Answer from the drawing. Dimensions are ordinates in mm from the lowest x, y and z of the part. A direction names the side the tool comes from. Round coordinates to 2 decimals unless told otherwise and drop trailing zeros. Order: outer loops, then holes, each group sorted by start corner. A loop starts at its lowest first (then second) coordinate and runs counter-clockwise, first axis right, second up. Notation, with made-up numbers: (12.25, 36.25) -> (67.25, 36.25) arc R17 cw to (67.25, 49.25) -> close; hole circle Ø8 at (32, 58.5). An arc over 180 degrees is marked (long way). Use a Markdown table: item, result. Add a question column.
Item 1: A flat-ended cylindrical pin translates along its axis: P1, Ø1, axis at x = 54, z = 20.5, coming from the +Y side. Find the tip coordinate at first contact, or state that the pin passes through.
Item 2: A cutting plane is placed at C-C, the plane x = 65.5. Determine the outline of the cut face in (y, z), plus the area to 3 significant figures.
Item 3: For a pull along Y with two mould halves and no side action, classify the marked faces 3, 4 and 5 as +Y half, -Y half, draft (parallel to the pull), parting line (faces both ways), or undercut.
Item 4: A tool of negligible diameter and unlimited length cuts with its end or side. For the marked faces 1 and 2, from which of +Z, -Z, +X, -X, +Y, -Y can it reach the whole face along a straight path? Write none if from no direction.
Item 5: A cutting plane is placed at B-B, the plane y = 71. Determine the outline of the cut face in (x, z), plus the area to 3 significant figures.
Item 6: Find the intervals of material crossed by L1, parallel to X at y = 55, z = 30.5; L2, parallel to Z at x = 6, y = 9; L3, parallel to X at y = 36, z = 25, in increasing order. Write a range as [from, to].
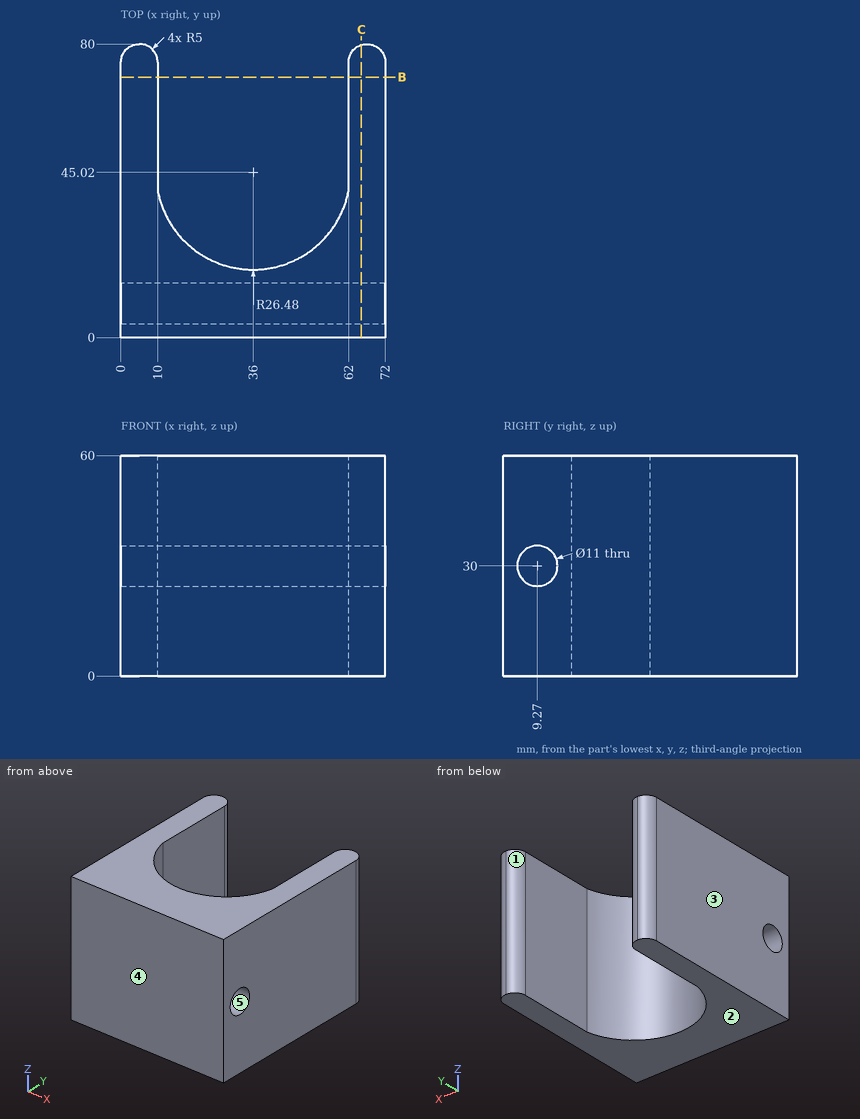
Reported:
| question | item | result |
|---|---|---|
| 1 | P1 | y = 26.07 |
| 2 | outline | (0, 0) -> (79.77, 0) -> (79.77, 60) -> (0, 60) -> close; hole circle Ø11 at (9.27, 30) |
| 2 | area | 4,690 mm² |
| 3 | face 3 | draft |
| 3 | face 4 | -Y half |
| 3 | face 5 | undercut |
| 4 | face 1 | +Z, -Z, +Y |
| 4 | face 2 | -Z, +X, -X, +Y, -Y |
| 5 | outline | (0, 0) -> (10, 0) -> (10, 60) -> (0, 60) -> close; (62, 0) -> (72, 0) -> (72, 60) -> (62, 60) -> close |
| 5 | area | 1,200 mm² |
| 6 | L1 | [0, 10], [62, 72] |
| 6 | L2 | [0, 24.51], [35.49, 60] |
| 6 | L3 | [0, 11.1], [60.9, 72] |
